The figure shows three views and two pictorial views of one solid part (mm, origin at its lowest corner). Answer the questions. Give positions to 0.01 mm unless a question says otherwise; leave off trailing zeros. Loops run counter-clockwise (first coordinate to the right, second up) from the corner with the lowest first, then second, coordinate; pieces in that order, holes last. Notation, with made-up numbers: (-10.5, 69.5) - (12.5, 69.5) arc R31 ccw to (12.5, 105.5) - close; hole circle Ø8 at (79, 81). An arc over 180 degrees is marked (long way). Use a Markdown table: item, result. Add a question column.
Item 1: This flat-tipped pin is pushed along its axis until it touches: P1, Ø0.6, axis at x = 69.5, y = 1, coming from the -Z side. Where does it stop, or does it pass through?
Item 2: Consider probe 1 along X at (y, z) = (0.15, 50); probe 2 along Z at (x, y) = (66, 0.8). Determine where each line is inside the solid, lowest interval first. Write a range as [from, to].
Item 3: A cutting plane is placed at B-B (z = 41). Determine the outline of the cut face in (x, y), plus the area to 3 significant figures.
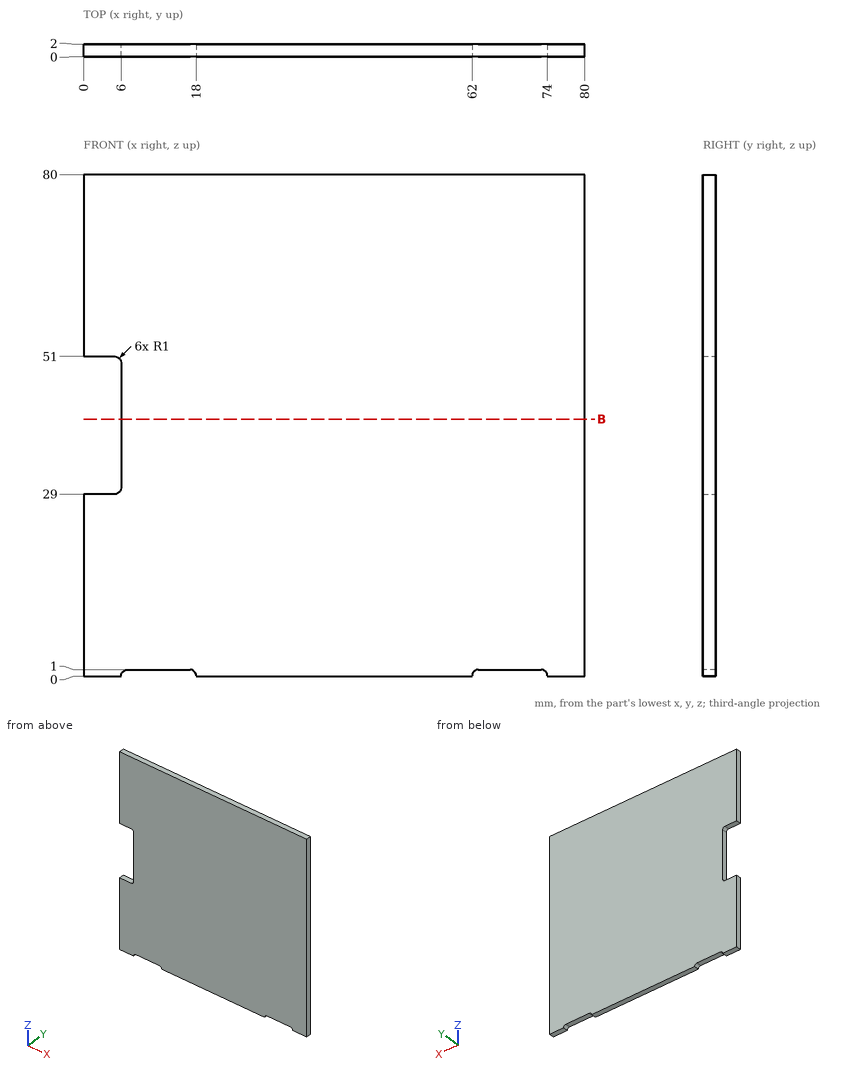
Geometry says:
| question | item | result |
|---|---|---|
| 1 | P1 | z = 1 |
| 2 | probe 1 | [6, 80] |
| 2 | probe 2 | [1, 80] |
| 3 | outline | (6, 0) - (80, 0) - (80, 2) - (6, 2) - close |
| 3 | area | 148 mm² |
